Work out the finished part from the listing and answer in its coordinate system (mm). Face numbers are marked on the shaded views. Round coordinates to 2 decimals unless told otherwise and drop trailing zeros. Write each loop counter-clockwise with the first axis right and the second up, starting at its lowest first coordinate (ties: lowest second). Pieces come first, ordered by that corner, then holes. Notation, with made-up numbers: (66, -4) - (70, -4) arc R8 cw to (70, 10) - close; hole circle Ø6 at (22.5, 18). An arc over 180 degrees is marked (long way). Answer as a JSON object with one key per item and string values.
```python
from build123d import *

# Parameters (mm, degrees)
SKETCH_1_R          = 2.25
EXTRUDE_2_DEPTH     = 25.5
SKETCH_7_W          = 2.4
SKETCH_7_H          = 2.4
CUT_EXTRUDE_3_DEPTH = 4.5
FILLET_2_R          = 2


with BuildPart() as part:
    # 草图1 → 凸台-拉伸2 (new body)
    with BuildSketch(Plane.XY):
        Circle(SKETCH_1_R)
    extrude(amount=EXTRUDE_2_DEPTH)

    # 草图7 → 切除-拉伸3 (cut)
    with BuildSketch(Plane.XY):
        Rectangle(SKETCH_7_W, SKETCH_7_H)
    extrude(amount=CUT_EXTRUDE_3_DEPTH, mode=Mode.SUBTRACT)

    # 圆角2
    fillet_2_edges = [part.edges().sort_by_distance(p)[0] for p in [
        (-2.25, 0, 25.5),
    ]]
    fillet(fillet_2_edges, radius=FILLET_2_R)


solid = part.part
```
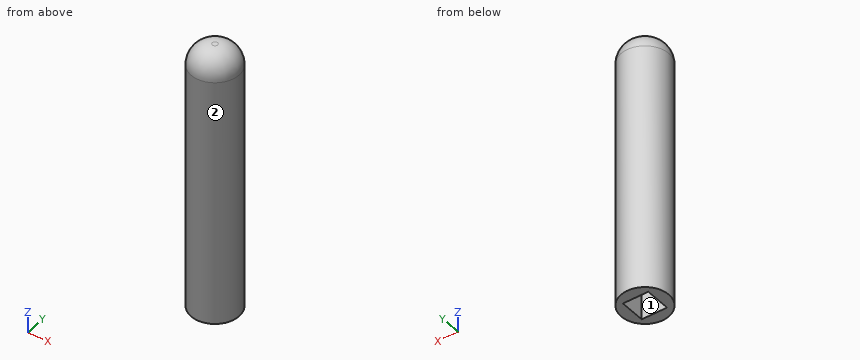
Item 1: Determine the mould class of the marked faces 1 and 2 for opening direction Y: pulls with the +Y half, pulls with the -Y half, needs draft (parallel to the pull), parting line crosses it, or undercut.
Results found:
{"face 1": "undercut", "face 2": "parting line crosses it"}
Item 2: A cutting plane is placed at A-A (z = 21). Write down the section's boundary in (x, y), and give its area (3 significant figures).
Results found:
{"outline": "circle Ø4.5 at (0, 0)", "area": "15.9 mm²"}
Item 3: This flat-tipped pin is pushed along its axis until it touches: P1, Ø0.7, axis at x = 0.5, y = 0, coming from the -Z side. Where does it stop, or does it pass through?
Results found:
{"P1": "z = 4.5"}
Item 4: Consider line 1 along X through (y, z) = (-1.9, 21); line 2 along Z through (x, y) = (0.3, 0); line 3 along X through (y, z) = (0.75, 3). Determine where each line is inside the solid, lowest interval first.
Results found:
{"line 1": "-1.21 to 1.21", "line 2": "4.5 to 25.5", "line 3": "-2.12 to -1.2, 1.2 to 2.12"}
